Check sheet for the modelled part. Datum: model origin and axes. Units: mm. A direction names the side the tool comes from. Give positions to 0.01 mm unless a question says otherwise; leave off trailing zeros. Loops run counter-clockwise (first coordinate to the right, second up) from the corner with the lowest first, then second, coordinate; pieces in that order, holes last. Notation, with made-up numbers: (28.25, 7.25) -> (32.25, 7.25) arc R34 ccw to (32.25, 45.25) -> close; hole circle Ø4 at (-21.5, 66). An arc over 180 degrees is marked (long way). Write each question's results on one line, items separated by ' | '. Start each with the question number.
Item 1: Cross-section at B-B on z = -7. Enter the section's corners in (x, y).
Item 2: Cross-section at A-A on x = 3.5. Enter the section's corners in (y, z), then the cut area to 3 significant figures.
Item 3: Cross-section at C-C on x = 34.5. Enter the section's corners in (y, z).
Item 4: Cross-section at D-D on z = 24. Enter the section's corners in (x, y).
Item 5: Scan lines: line 1 along Z through (x, y) = (3.5, 8.7); line 2 along Y through (x, z) = (-25, -73); line 3 along Z through (x, y) = (31, 94). Record each from-to range of solid material in increasing order.
Item 6: Mould release check, pull along Z, two halves, no side actions. Record for faces 6 (the face through (25, 157, -94)), 7 (the face through (-40, 118, -45)), 8 (the face through (-45, 110, 50)), 9 (the face through (1, 8, 45.5)): pulls with the +Z half, pulls with the -Z half, needs draft (parallel to the pull), parting line crosses it, or undercut.
Item 7: Gauge pin test, flat ends, axial feed: pin 1 Ø19 at (y, z) = (145.5, -53) entering from +X; pin 2 Ø5 at (y, z) = (212, -88) entering from -X; pin 3 Ø6 at (y, z) = (137, -45.5) entering from -X. Record the tip position at first contact, or that the pin passes through.
Item 8: Access from +Z, -Z, +X, -X, +Y, -Y to the whole of each face (thin tool, end or side, straight path). Record for faces 1 (the face through (40.5, 8, 2)), 2 (the face through (40, 118, -45)), 3 (the face through (-1, 5, -105)), 4 (the face through (-18, 158, -94)), 5 (the face through (35, 118, -50)).
from build123d import *

# Parameters (mm, degrees)
SKETCH1_W           = 100
SKETCH1_H           = 100
BOSS_EXTRUDE1_DEPTH = 10
BOSS_EXTRUDE2_DEPTH = 220
SKETCH4_W           = 100
SKETCH4_H           = 40
BOSS_EXTRUDE3_DEPTH = 10
SKETCH5_W           = 100
SKETCH5_H           = 140
BOSS_EXTRUDE4_DEPTH = 8
CUT_EXTRUDE2_DEPTH  = 11
SKETCH7_W           = 8
SKETCH7_H           = 8
BOSS_EXTRUDE5_DEPTH = 220
CUT_EXTRUDE3_DEPTH  = 5
CUT_EXTRUDE4_REACH  = 7
SKETCH9_W           = 40
SKETCH9_H           = 20
SKETCH11_W          = 100
SKETCH11_H          = 15
BOSS_EXTRUDE6_DEPTH = 10
SKETCH12_R          = 3
CUT_EXTRUDE5_DEPTH  = 2
BOSS_EXTRUDE7_DEPTH = 228
SKETCH14_W          = 35.5
SKETCH14_H          = 4
SKETCH14_W_2        = 28.5
BOSS_EXTRUDE8_DEPTH = 8


with BuildPart() as part:
    # Sketch1 → Boss-Extrude1 (new body)
    with BuildSketch(Plane(origin=(0, 0, 0), x_dir=(1, 0, 0), z_dir=(0, 1, 0))):
        Rectangle(SKETCH1_W, SKETCH1_H)
    extrude(amount=BOSS_EXTRUDE1_DEPTH)

    # Sketch3 → Boss-Extrude2 (add)
    with BuildSketch(Plane(origin=(0, 10, 0), x_dir=(1, 0, 0), z_dir=(0, 1, 0))):
        Polygon((-40, 40), (-40, 50), (-30, 50), (-30, 47.7), (-37, 47.7), (-37, 42.3), (-30, 42.3), (-30, 40), align=None)
        Polygon((30, 42.3), (30, 40), (40, 40), (40, 50), (30, 50), (30, 47.7), (37, 47.7), (37, 42.3), align=None)
    extrude(amount=BOSS_EXTRUDE2_DEPTH)

    # Sketch4 → Boss-Extrude3 (add)
    with BuildSketch(Plane(origin=(0, 0, 0), x_dir=(1, 0, 0), z_dir=(0, 1, 0))):
        with Locations((0, 70)):
            Rectangle(SKETCH4_W, SKETCH4_H)
    extrude(amount=BOSS_EXTRUDE3_DEPTH)

    # Sketch5 → Boss-Extrude4 (add)
    with BuildSketch(Plane(origin=(0, 230, 0), x_dir=(1, 0, 0), z_dir=(0, 1, 0))):
        with Locations((0, 20)):
            Rectangle(SKETCH5_W, SKETCH5_H)
    extrude(amount=BOSS_EXTRUDE4_DEPTH)

    # Sketch6 → Cut-Extrude2 (cut)
    with BuildSketch(Plane(origin=(0, 238, 0), x_dir=(1, 0, 0), z_dir=(0, 1, 0))):
        Polygon((-4.5, 30), (30, 30), (30, 90), (-4.5, 90), (-14.5, 90), (-14.5, 30), align=None)
    extrude(amount=-CUT_EXTRUDE2_DEPTH, mode=Mode.SUBTRACT)

    # Sketch7 → Boss-Extrude5 (add)
    with BuildSketch(Plane(origin=(0, 10, 0), x_dir=(1, 0, 0), z_dir=(0, 1, 0))):
        with Locations((-46, -46)):
            Rectangle(SKETCH7_W, SKETCH7_H)
        with Locations((46, -46)):
            Rectangle(SKETCH7_W, SKETCH7_H)
    extrude(amount=BOSS_EXTRUDE5_DEPTH)

    # Sketch8 → Cut-Extrude3 (cut)
    with BuildSketch(Plane(origin=(0, 10, 0), x_dir=(1, 0, 0), z_dir=(0, 1, 0))):
        Polygon((30, 40), (40.5, 40), (40.5, -45.5), (-40.5, -45.5), (-40.5, 40), (-30, 40), (-30, 50.5), (30, 50.5), align=None)
    extrude(amount=-CUT_EXTRUDE3_DEPTH, mode=Mode.SUBTRACT)

    # Sketch9 → Cut-Extrude4 (cut, up to next)
    with BuildSketch(Plane(origin=(0, 5, 0), x_dir=(1, 0, 0), z_dir=(0, 1, 0)), mode=Mode.PRIVATE) as cut_extrude4_sk1:
        Rectangle(SKETCH9_W, SKETCH9_H)
    cut_extrude4_tool1 = extrude(cut_extrude4_sk1.sketch, amount=-CUT_EXTRUDE4_REACH, mode=Mode.PRIVATE) & part.part
    add(cut_extrude4_tool1.solids().sort_by_distance((0, 5, 0))[0], mode=Mode.SUBTRACT)

    # Sketch11 → Boss-Extrude6 (add)
    with BuildSketch(Plane(origin=(0, 0, 0), x_dir=(1, 0, 0), z_dir=(0, 1, 0))):
        with Locations((0, 97.5)):
            Rectangle(SKETCH11_W, SKETCH11_H)
    extrude(amount=BOSS_EXTRUDE6_DEPTH)

    # Sketch12 → Cut-Extrude5 (cut)
    with BuildSketch(Plane(origin=(0, 10, 0), x_dir=(1, 0, 0), z_dir=(0, 1, 0))):
        with Locations((3.5, 96.967812545)):
            Circle(SKETCH12_R)
    extrude(amount=-CUT_EXTRUDE5_DEPTH, mode=Mode.SUBTRACT)

    # Sketch13 → Boss-Extrude7 (add)
    with BuildSketch(Plane(origin=(0, 10, 0), x_dir=(1, 0, 0), z_dir=(0, 1, 0))):
        Polygon((21.5, 92), (23.5, 92), (23.5, 94), (25.5, 94), (25.5, 90), (21.5, 90), align=None)
        Polygon((-14.5, 92), (-16.5, 92), (-16.5, 94), (-18.5, 94), (-18.5, 90), (-14.5, 90), align=None)
    extrude(amount=BOSS_EXTRUDE7_DEPTH)

    # Sketch14 → Boss-Extrude8 (add)
    with BuildSketch(Plane(origin=(0, 238, 0), x_dir=(1, 0, 0), z_dir=(0, 1, 0))):
        with Locations((-32.25, 92)):
            Rectangle(SKETCH14_W, SKETCH14_H)
        with Locations((35.75, 92)):
            Rectangle(SKETCH14_W_2, SKETCH14_H)
    extrude(amount=-BOSS_EXTRUDE8_DEPTH)


solid = part.part
Answer sheet:
1) outline: (-50, 0) -> (-20, 0) -> (-20, 5) -> (-40.5, 5) -> (-40.5, 10) -> (-50, 10) -> close; (-50, 230) -> (50, 230) -> (50, 238) -> (-50, 238) -> close; (20, 0) -> (50, 0) -> (50, 10) -> (40.5, 10) -> (40.5, 5) -> (20, 5) -> close
2) outline: (0, -105) -> (10, -105) -> (10, -99.97) -> (8, -99.97) -> (8, -93.97) -> (10, -93.97) -> (10, -50.5) -> (5, -50.5) -> (5, -10) -> (0, -10) -> close; (0, 10) -> (5, 10) -> (5, 45.5) -> (10, 45.5) -> (10, 50) -> (0, 50) -> close; (230, -30) -> (238, -30) -> (238, 50) -> (230, 50) -> close | area: 1,600 mm²
3) outline: (0, -105) -> (10, -105) -> (10, -50) -> (230, -50) -> (230, -94) -> (238, -94) -> (238, 50) -> (230, 50) -> (230, -40) -> (5, -40) -> (5, 45.5) -> (10, 45.5) -> (10, 50) -> (0, 50) -> close; hole (10, -47.7) -> (230, -47.7) -> (230, -42.3) -> (10, -42.3) -> close
4) outline: (-50, 0) -> (50, 0) -> (50, 10) -> (40.5, 10) -> (40.5, 5) -> (-40.5, 5) -> (-40.5, 10) -> (-50, 10) -> close; (-50, 230) -> (50, 230) -> (50, 238) -> (-50, 238) -> close
5) line 1: z = -105 to -99.97, -93.97 to -50.5, 45.5 to 50 | line 2: y = 0 to 10, 230 to 238 | line 3: z = -50 to -47.7, -42.3 to -40
6) face 6: pulls with the -Z half | face 7: needs draft | face 8: pulls with the +Z half | face 9: undercut
7) pin 1: stops at x = 40 | pin 2: stops at x = -18.5 | pin 3: stops at x = -40
8) face 1: none | face 2: +Z, -Z, +X | face 3: -Z, +X, -X, +Y, -Y | face 4: -Z, +X, -X, +Y | face 5: -Z, +X, -X
